Design review of the part built by this model. Coordinates are the model's own, in mm. A direction names the side the tool comes from. Coordinates: 2 decimals unless noted, no trailing zeros. Write each loop counter-clockwise with the first axis right and the second up, starting at its lowest first coordinate (ties: lowest second). Pieces come first, ordered by that corner, then holes.
Q1. Take a section at B-B (x = 0). Give the boundary of the cut face in (y, z) (3 decimals).
Q2. Insertion check: pin 1 (2 mm diameter, centred on y = 1, z = -4, fed in from +X); pin 2 (1.5 mm diameter, centred on y = -1.5, z = -0.5, fed in from +X); pin 3 (2 mm diameter, centred on x = 1, y = -1, fed in from -Z). Each pin has a flat end and moves straight along its axis. Give the tip position at first contact, or say it passes through.
Q3. Machinability: for faces 5 (the flat face through (-5, 0, -7)), 6 (the flat face through (-2, 1, 0)), which of the approach directions +Z, -Z, +X, -X, +Y, -Y give a long, thin tool a straight path to every point of the face, cutting with its end or side? Answer none if there is none.
Q4. Take a section at C-C (z = -0.25). Give the boundary of the cut face in (x, y).
Q5. Take a section at D-D (y = -1.25). Give the boundary of the cut face in (x, z).
Q6. Take a section at A-A (y = 0). Give the boundary of the cut face in (x, z) (3 decimals).
Q7. Mouldability with a two-part tool opening along Y and no side actions: class faces 1 (the cylindrical face through (1.56, -0.49, 0.99)), 2 (the flat face through (2.5, 0, 1)), 3 (the cylindrical face through (-5.715, 3.199, -2.563)), 4 (the cylindrical face through (-5.715, -3.199, -2.437)) as pulls with the +Y half, pulls with the -Y half, needs draft (parallel to the pull), parting line crosses it, or undercut.
Q8. For probe 1 along X at (y, z) = (0.75, -1.75); probe 2 along Z at (x, y) = (1.75, 1.5); probe 3 along X at (y, z) = (-0.5, 1.5), list the stretches that pass through material, from the lowest coordinate up.
Autodesk Inventor part; units mm, degrees
ref_plane "YZ Plane" through (0, 0, 0) normal (1, 0, 0) x (0, 1, 0)
ref_plane "XZ Plane" through (0, 0, 0) normal (0, 1, 0) x (-1, 0, 0)
ref_plane "XY Plane" through (0, 0, 0) normal (0, 0, 1) x (1, 0, 0)
sketch "スケッチ1" plane through (0, 0, 0) normal (0, 0, 1) x (1, 0, 0)
  circle A0 centre (0, 0) radius 1.635
  line L0 (-6, -3.5) -> (2.5, -3.5)
  line L1 (2.5, -3.5) -> (2.5, 3.5)
  line L2 (2.5, 3.5) -> (-6, 3.5)
  line L3 (-6, 3.5) -> (-6, -3.5)
  line L4 (-6, -3.5) -> (2.5, 3.5) construction
  line L5 (2.5, -3.5) -> (-6, 3.5) construction
  line L6 (-6, 0) -> (2.5, 0) construction
  line L7 (-4, 3.5) -> (-4, -3.5)
  point P0 (-1.75, 0)
  dimension "d0" = 3.27
  dimension "d1" = 7
  dimension "d2" = 2.5
  dimension "d3" = 6
  dimension "d6" = 2
extrude "押し出し1" add sketch "スケッチ1" along normal blind 2
extrude "押し出し2" add sketch "スケッチ1" against normal blind 7 contours L3 L2 L7 L0
fillet "フィレット1" radius 3 2 edges at (2.5, 3.5, 1) (2.5, -3.5, 1)
fillet "フィレット2" radius 1 2 edges at (-6, -3.5, -2.5) (-6, 3.5, -2.5)
properties part number "guide_link"
Response:
1. outline: (-3.458, 0) - (-1.635, 0) - (-1.635, 2) - (-3.458, 2) - close; (1.635, 0) - (3.458, 0) - (3.458, 2) - (1.635, 2) - close
2. pin 1: stops at x = -4
2. pin 2: stops at x = 2.47
2. pin 3: stops at z = 0
3. face 5: -Z, +X, -X, +Y, -Y
3. face 6: -Z, +X, +Y, -Y
4. outline: (-6, -2.5) arc R1 ccw to (-5, -3.5) - (-4, -3.5) - (-4, 3.5) - (-5, 3.5) arc R1 ccw to (-6, 2.5) - close
5. outline: (-6, -7) - (-4, -7) - (-4, 0) - (-1.05, 0) - (-1.05, 2) - (-6, 2) - close; (1.05, 0) - (2.4, 0) - (2.4, 2) - (1.05, 2) - close
6. outline: (-6, -7) - (-4, -7) - (-4, 0) - (-1.635, 0) - (-1.635, 2) - (-6, 2) - close; (1.635, 0) - (2.5, 0) - (2.5, 2) - (1.635, 2) - close
7. face 1: undercut
7. face 2: needs draft
7. face 3: pulls with the +Y half
7. face 4: pulls with the -Y half
8. probe 1: x = -6 to -4
8. probe 2: z = 0 to 2
8. probe 3: x = -6 to -1.56, 1.56 to 2.5
